```python
from build123d import *

# Parameters (mm, degrees)
ESBO_O4_R             = 1.75
CORTE_EXTRUS_O1_DEPTH = 2


with BuildPart() as part:
    # Esboço2 → Revolução1 (revolve)
    with BuildSketch(Plane.XY):
        with BuildLine():
            Line((1.25, 6.25), (13.75, 6.25))
            Line((13.75, 6.25), (13.75, 10))
            Line((13.75, 10), (12.5, 15))
            Line((12.5, 15), (12.5, 20))
            Line((12.5, 20), (15, 25))
            Line((15, 25), (15, 32))
            Line((15, 32), (12.5, 32))
            Line((12.5, 32), (12.5, 29))
            ThreePointArc((12.5, 29), (11.914213562, 27.585786438), (10.5, 27))
            Line((10.5, 27), (4.5, 27))
            ThreePointArc((4.5, 27), (3.085786438, 27.585786438), (2.5, 29))
            Line((2.5, 29), (2.5, 32))
            Line((2.5, 32), (0, 32))
            Line((0, 32), (0, 25))
            Line((0, 25), (2.5, 20))
            Line((2.5, 20), (2.5, 15))
            Line((2.5, 15), (1.25, 10))
            Line((1.25, 10), (1.25, 6.25))
        make_face()
    revolve(axis=Axis((0, 0, 0), (1, 0, 0)))

    # Esboço4 → Corte-extrusão1 (cut)
    with BuildSketch(Plane(origin=(15, 0, 0), x_dir=(0, 0, -1), z_dir=(1, 0, 0))):
        with Locations((0, 28)):
            Circle(ESBO_O4_R)
    extrude(amount=-CORTE_EXTRUS_O1_DEPTH, mode=Mode.SUBTRACT)


solid = part.part
```
Geometry: final body of the model. Coordinates: model frame, mm. A direction names the side the tool comes from. Round coordinates to 2 decimals unless told otherwise and drop trailing zeros. Order: outer loops, then holes, each group sorted by start corner. A loop starts at its lowest first (then second) coordinate and runs counter-clockwise, first axis right, second up. Notation, with made-up numbers: (86.25, 27) -> (106.25, 27) arc R12 ccw to (106.25, 39) -> close; hole circle Ø2 at (-15.75, 68). An arc over 180 degrees is marked (long way). Use one line per item in the form item = value. Start each with the question number.
1. Reachability of faces 1 (the face through (2.5, 3, 15)), 2 (the face through (7.46, -5.85, -26.36)), 3 (the face through (14.01, 26.45, -0.81)) from +Z, -Z, +X, -X, +Y, -Y: full face, straight path, thin tool, end or side. Return the list, or none.
2. Line query: probe 1 along X at (y, z) = (5, 28.5); probe 2 along Z at (x, y) = (4.5, 0); probe 3 along X at (y, z) = (-5.5, -7). Output: solid intervals per line, ascending.
3. Cut plane A-A (x = 6.25). Return the cut outline in (y, z), then the cut area to 3 significant figures.
4. Draft query along Y for faces 4 (the face through (1.23, -6.94, -31.24)), 5 (the face through (1.25, 4, 5)), 6 (the face through (0, -19.1, -16.4)), 7 (the face through (13, 28, 0)). Return one class per face: pulls with the +Y half, pulls with the -Y half, needs draft (parallel to the pull), parting line crosses it, or undercut.
5. Pin query (flat end, axial travel): pin 1 Ø3 at (y, z) = (28, 0) entering from +X; pin 2 Ø1.5 at (x, z) = (7.5, -3) entering from +Y; pin 3 Ø4 at (x, z) = (2.5, -3) entering from +Y. Return the tip coordinate at first contact, or that it passes through.
Solution:
q1.face_1 = -X
q1.face_2 = none
q1.face_3 = +X
q2.probe_1 = 0 to 2.5, 12.5 to 15
q2.probe_2 = -27 to -6.25, 6.25 to 27
q2.probe_3 = 1.25 to 13.75
q3.outline = circle Ø54 at (0, 0); hole circle Ø12.5 at (0, 0)
q3.area = 2,170 mm^2
q4.face_4 = parting line crosses it
q4.face_5 = undercut
q4.face_6 = needs draft
q4.face_7 = undercut
q5.pin_1 = 13
q5.pin_2 = 26.91
q5.pin_3 = 31.98
